Read the model definition and answer for the solid it produces. Units are mm, in the model's axes. A direction names the side the tool comes from. Coordinates: 2 decimals unless noted, no trailing zeros. Order: outer loops, then holes, each group sorted by start corner. A loop starts at its lowest first (then second) coordinate and runs counter-clockwise, first axis right, second up. Notation, with made-up numbers: (-4, -27.5) - (27, -27.5) arc R13 cw to (27, -6.5) - close; hole circle Ø9 at (-24, 65.25). An arc over 180 degrees is marked (long way). Use one line per item in the form item = value. Start each with the question number.
from build123d import *

# Parameters (mm, degrees)
F0_W     = 750
F0_H     = 400
F1_DEPTH = 700
F2_W     = 300
F2_H     = 600
F3_DEPTH = 700


with BuildPart() as f1:
    # F0 (on Top) → F1 (new body)
    with BuildSketch(Plane.XY):
        Rectangle(F0_W, F0_H)
    extrude(amount=F1_DEPTH)

    # F2 (on face) → F3 (cut, through all)
    with BuildSketch(Plane.YZ.offset(375)):
        with Locations((0, 350)):
            Rectangle(F2_W, F2_H)
    extrude(amount=-F3_DEPTH, mode=Mode.SUBTRACT)

    # F4 (on Front) → F5 (revolve)
    with BuildSketch(Plane.XZ):
        with BuildLine():
            Line((0, 1100), (-100, 1100))
            add(Edge.make_bspline(
                [(-100, 1100), (-74.9264732003, 1074.5007991791), (-52.4668861873, 995.3000976798), (-167.4321274896, 851.7977207352), (-48.4324080123, 747.3342060696), (-88.7868594089, 716.1834569746), (-125, 700)],
                knots=[0, 0, 0, 0, 0.2434136268, 0.5448860938, 0.7983932105, 1, 1, 1, 1], degree=3))
            Line((-125, 700), (0, 700))
            Line((0, 700), (0, 1100))
        make_face()
    revolve(axis=Axis((0, 0, 550), (0, 0, 1)))


solid = f1.part
Q1. A cutting plane is placed at B-B (z = 576.5). Give the vertices of the cut face in (x, y).
Q2. For a pull along Y with two mould halves and no side action, classify faces 3 (the flat face through (-325, -2, 354)), 4 (the flat face through (375, -181, 345)), 5 (the flat face through (-5, 200, 345)), 6 (the flat face through (-5, -200, 345)) as +Y half, -Y half, draft (parallel to the pull), parting line (faces both ways), or undercut.
Q3. Given P1, Ø1.5, axis at x = -197.5, y = -81, coming from the +Z side; P2, Ø3, axis at y = -17.5, z = 608, coming from the +X side; P3, Ø1.5, axis at x = -90.5, z = 813.5, coming from the -Y side, each flat-ended and moving along its own axis, determine where each tip first touches the part or whether it passes through.
Q4. Consider probe 1 along Z at (x, y) = (174.5, -3); probe 2 along Y at (x, z) = (282, 616.5); probe 3 along Z at (x, y) = (-32, 7). Determine where each line is inside the solid, lowest interval first.
Q5. A cutting plane is placed at A-A (x = -253). Give the vertices of the cut face in (y, z).
Q6. A cutting plane is placed at D-D (x = -88.5). Give the number of separate pieces and of enclosed holes in the cut face, then the cut area to 3 significant figures.
Q7. Which of the six approach directions +Z, -Z, +X, -X, +Y, -Y give full straight-line access (tool end or side, diameter ignored) to faces 1 (the flat face through (30, -2, 650)), 2 (the flat face through (-375, -3, 345))?
Q8. A cutting plane is placed at C-C (y = 176). Give the vertices of the cut face in (x, z).
Result sheet:
q1.outline = (-375, -200) - (375, -200) - (375, -150) - (-325, -150) - (-325, 150) - (375, 150) - (375, 200) - (-375, 200) - close
q2.face_3 = undercut
q2.face_4 = draft
q2.face_5 = +Y half
q2.face_6 = -Y half
q3.P1 = 700
q3.P2 = -325
q3.P3 = -66.93
q4.probe_1 = 0 to 50, 650 to 700
q4.probe_2 = -200 to -150, 150 to 200
q4.probe_3 = 0 to 50, 650 to 1100
q5.outline = (-200, 0) - (200, 0) - (200, 700) - (-200, 700) - close; hole (-150, 50) - (150, 50) - (150, 650) - (-150, 650) - close
q6.separate_pieces = 3
q6.enclosed_holes = 1
q6.area = 127,000 mm^2
q7.face_1 = +X
q7.face_2 = +Z, -Z, -X, +Y, -Y
q8.outline = (-375, 0) - (375, 0) - (375, 700) - (-375, 700) - close
